from build123d import *

# Parameters (mm, degrees)
BOSS_EXTRUDE1_DEPTH = 8.89
CHAMFER1_SIZE       = 2.54
HOLE1_AT_2_COUNT    = 2
HOLE1_AT_2_PITCH    = 7.62


with BuildPart() as part:
    # Sketch1 → Boss-Extrude1 (new body)
    with BuildSketch(Plane.XY):
        with BuildLine():
            Line((6.020580432, 9.158318359), (-7.695419568, 9.158318359))
            Line((-7.695419568, 9.158318359), (-7.695419568, 0.268318359))
            ThreePointArc((-7.695419568, 0.268318359), (-0.837419568, -6.589681641), (6.020580432, 0.268318359))
            Line((6.020580432, 0.268318359), (6.020580432, 9.158318359))
        make_face()
    extrude(amount=-BOSS_EXTRUDE1_DEPTH)

    # Chamfer1
    chamfer1_edges = [part.edges().sort_by_distance(p)[0] for p in [
        (-0.837419568, -6.589681641, -8.89),
        (6.020580432, 4.713318359, -8.89),
        (-7.695419568, 4.713318359, -8.89),
    ]]
    chamfer(chamfer1_edges, length=CHAMFER1_SIZE)

    # Sketch3 → Hole1 (revolve, cut)
    with BuildSketch(Plane(origin=(2.972580432, 9.158318359, -3.175), x_dir=(0, 0, 1), z_dir=(1, 0, 0))):
        Polygon((0, 0), (0, 3.81), (2.5273, 3.81), (2.6543, 0), align=None)
    hole1 = revolve(axis=Axis((2.972580432, -100.841681641, -3.175), (0, 1, 0)), mode=Mode.SUBTRACT)

    # Hole1 at 2: Hole1 ×2
    with Locations(*[(-i * HOLE1_AT_2_PITCH, 0, 0) for i in range(1, HOLE1_AT_2_COUNT)]):
        add(hole1, mode=Mode.SUBTRACT)


solid = part.part
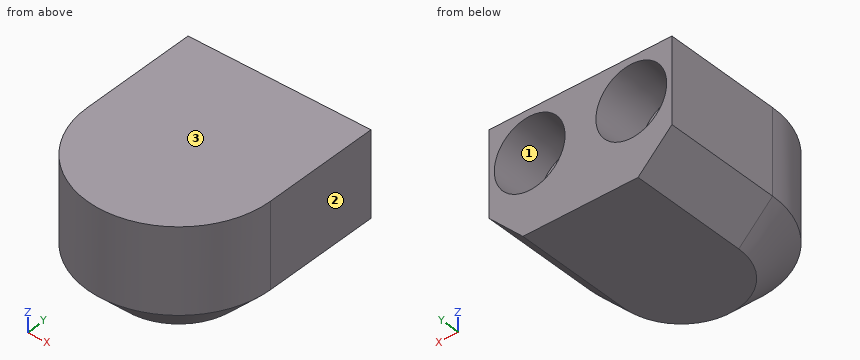
Design review of the part built by this model. Coordinates are the model's own, in mm. Face numbers are marked on the shaded views. Round coordinates to 2 decimals unless told otherwise and drop trailing zeros. Write each loop counter-clockwise with the first axis right and the second up, starting at its lowest first coordinate (ties: lowest second). Pieces come first, ordered by that corner, then holes. Notation, with made-up numbers: (38.25, -36.5) -> (44.25, -36.5) arc R13 cw to (44.25, -17.5) -> close; hole circle Ø8 at (60, 47). An arc over 180 degrees is marked (long way). One line per question, with ' | ' between items.
(1) Draft analysis for pull direction X (two halves, no side actions). For the marked faces 1, 2 and 3, state which applies: released by +X, released by -X, zero draft, split by the parting line, or undercut.
Result sheet:
face 1: undercut | face 2: released by +X | face 3: zero draft
(2) Insertion check: P1, Ø2.5, axis at x = -4, z = -3.5, coming from the +Y side; P2, Ø1, axis at y = -2.5, z = -1, coming from the +X side. Each pin has a flat end and moves straight along its axis. Give the tip position at first contact, or say it passes through.
Result sheet:
P1: y = 5.35 | P2: x = 5.63
(3) Wall thickness on line 1 (X direction, y = 7, z = -3.25); line 2 (X direction, y = 5.5, z = -5); line 3 (Z direction, x = -4, y = 7.25): over which ranges is each line inside the solid? List them lowest first. Write a range as [from, to].
Result sheet:
line 1: [-7.7, -7.23], [-2.07, 0.39], [5.55, 6.02] | line 2: [-7.7, -6.4], [-2.89, 1.22], [4.73, 6.02] | line 3: [-8.89, -5.68], [-0.67, 0]
(4) Take a section at B-B, the plane y = 3. State the section outline as (x, z) points, and give its area (3 significant figures).
Result sheet:
outline: (-7.7, -6.35) -> (-5.16, -8.89) -> (3.48, -8.89) -> (6.02, -6.35) -> (6.02, 0) -> (-7.7, 0) -> close | area: 115 mm2
(5) Take a section at A-A, the plane y = 7.5. State the section outline as (x, z) points (3 decimals).
Result sheet:
outline: (-7.695, -6.35) -> (-5.155, -8.89) -> (3.481, -8.89) -> (6.021, -6.35) -> (6.021, 0) -> (-7.695, 0) -> close; hole circle Ø5.198 at (-4.647, -3.175); hole circle Ø5.198 at (2.973, -3.175)
